Work out the finished part from the listing and answer in its coordinate system (mm). A direction names the side the tool comes from. Give positions to 0.01 mm unless a question says otherwise; leave off trailing zeros. Loops run counter-clockwise (first coordinate to the right, second up) from the corner with the lowest first, then second, coordinate; pieces in that order, holes last. Notation, with made-up numbers: (22, 25) - (67, 25) arc R14 ccw to (67, 45) - close; hole circle Ø4 at (-17, -11.75). An arc over 180 degrees is marked (long way). Use CSV: the item, a comma, the result in double quotes.
from build123d import *

# Parameters (mm, degrees)
F0_W     = 76
F0_H     = 190
F0_R     = 3.5
F0_R_2   = 20
F1_DEPTH = 7


# Not quite as in the source:
# - a feature names something its author has since deleted; it is built from what else it names


with BuildPart() as f1:
    # F0 (on Top) → F1 (new body)
    with BuildSketch(Plane.XY):
        with Locations((0, 60)):
            Rectangle(F0_W, F0_H)
        with Locations((-23.57, -23.57)):
            Circle(F0_R, mode=Mode.SUBTRACT)
        with Locations((-23.57, 23.57)):
            Circle(F0_R, mode=Mode.SUBTRACT)
        Circle(F0_R_2, mode=Mode.SUBTRACT)
        with Locations((23.57, -23.57)):
            Circle(F0_R, mode=Mode.SUBTRACT)
        with Locations((23.57, 23.57)):
            Circle(F0_R, mode=Mode.SUBTRACT)
        with BuildLine():
            Line((-27.07, 86.43), (-27.07, 96.43))
            ThreePointArc((-27.07, 96.43), (-23.5699996641, 99.93), (-20.07, 96.4299993282))
            Line((-20.07, 96.4299993282), (-20.07, 86.4299993282))
            ThreePointArc((-20.07, 86.4299993282), (-23.5700003359, 82.93), (-27.07, 86.43))
        make_face(mode=Mode.SUBTRACT)
        with BuildLine():
            Line((-27.07, 133.57), (-27.07, 143.57))
            ThreePointArc((-27.07, 143.57), (-23.5699996641, 147.07), (-20.07, 143.5699993282))
            Line((-20.07, 143.5699993282), (-20.07, 133.5699993282))
            ThreePointArc((-20.07, 133.5699993282), (-23.5700003359, 130.07), (-27.07, 133.57))
        make_face(mode=Mode.SUBTRACT)
        with BuildLine():
            Line((20.07, 86.43), (20.07, 96.43))
            ThreePointArc((20.07, 96.43), (23.5700003359, 99.93), (27.07, 96.4299993282))
            Line((27.07, 96.4299993282), (27.07, 86.4299993282))
            ThreePointArc((27.07, 86.4299993282), (23.5699996641, 82.93), (20.07, 86.43))
        make_face(mode=Mode.SUBTRACT)
        with BuildLine():
            Line((-20, 110), (-20, 120))
            ThreePointArc((-20, 120), (1.2657e-06, 140), (20, 119.9999974687))
            Line((20, 119.9999974687), (20, 109.9999974687))
            ThreePointArc((20, 109.9999974687), (-1.2657e-06, 90), (-20, 110))
        make_face(mode=Mode.SUBTRACT)
        with BuildLine():
            Line((20.07, 133.57), (20.07, 143.57))
            ThreePointArc((20.07, 143.57), (23.5700003359, 147.07), (27.07, 143.5699993282))
            Line((27.07, 143.5699993282), (27.07, 133.5699993282))
            ThreePointArc((27.07, 133.5699993282), (23.5699996641, 130.07), (20.07, 133.57))
        make_face(mode=Mode.SUBTRACT)
    extrude(amount=F1_DEPTH)


solid = f1.part
Item 1: A cutting plane is placed at B-B on x = -23.57. Determine the outline of the cut face in (y, z), and give its area (3 significant figures).
Determined:
outline,"(-35, 0) - (-27.07, 0) - (-27.07, 7) - (-35, 7) - close; (-20.07, 0) - (20.07, 0) - (20.07, 7) - (-20.07, 7) - close; (27.07, 0) - (82.93, 0) - (82.93, 7) - (27.07, 7) - close; (99.93, 0) - (130.07, 0) - (130.07, 7) - (99.93, 7) - close; (147.07, 0) - (155, 0) - (155, 7) - (147.07, 7) - close"
area,"994 mm²"
Item 2: The mould has two halves that part along X. Classify faces 3 (the flat face through (-1, 61, 7)), 4 (the flat face through (27.07, 91, 3)), 5 (the flat face through (38, 59, 3)): pulls with the +X half, pulls with the -X half, needs draft (parallel to the pull), parting line crosses it, or undercut.
Determined:
face 3,"needs draft"
face 4,"undercut"
face 5,"pulls with the +X half"
Item 3: A cutting plane is placed at C-C on y = 0. Determine the outline of the cut face in (x, z), and give its area (3 significant figures).
Determined:
outline,"(-38, 0) - (-20, 0) - (-20, 7) - (-38, 7) - close; (20, 0) - (38, 0) - (38, 7) - (20, 7) - close"
area,"252 mm²"
Item 4: Given P1, Ø1.5, axis at x = 11, y = 13.5, coming from the -Z side, flat-ended and moving along its own axis, determine where the tip first touches the part or whether it passes through.
Determined:
P1,"passes through"
Item 5: A cutting plane is placed at D-D on x = 0. Determine the outline of the cut face in (y, z).
Determined:
outline,"(-35, 0) - (-20, 0) - (-20, 7) - (-35, 7) - close; (20, 0) - (90, 0) - (90, 7) - (20, 7) - close; (140, 0) - (155, 0) - (155, 7) - (140, 7) - close"
Item 6: A cutting plane is placed at A-A on y = -23.57. Determine the outline of the cut face in (x, z).
Determined:
outline,"(-38, 0) - (-27.07, 0) - (-27.07, 7) - (-38, 7) - close; (-20.07, 0) - (20.07, 0) - (20.07, 7) - (-20.07, 7) - close; (27.07, 0) - (38, 0) - (38, 7) - (27.07, 7) - close"
Item 7: For faces 1 (the flat face through (-20.07, 91, 3)), 2 (the flat face through (-1, 61, 0)), determine the directions among +Z, -Z, +X, -X, +Y, -Y from which every point of the face is accessible in a straight line to the end or side of a thin tool.
Determined:
face 1,"+Z, -Z"
face 2,"-Z, +X, -X, +Y, -Y"
Item 8: Find the intervals of material crossed by line 1 (Y direction, x = 0, z = 4.25); line 2 (X direction, y = 86, z = 0.75); line 3 (Y direction, x = -24, z = 3.5), in increasing order.
Determined:
line 1,"y = -35 to -20, 20 to 90, 140 to 155"
line 2,"x = -38 to -27.04, -20.1 to 20.1, 27.04 to 38"
line 3,"y = -35 to -27.04, -20.1 to 20.1, 27.04 to 82.96, 99.9 to 130.1, 147.04 to 155"
